Source: CAD feature listing. Evaluate the final solid. Frame: model axes, mm. A direction names the side the tool comes from. Give positions to 0.01 mm unless a question says otherwise; leave off trailing zeros. Order: outer loops, then holes, each group sorted by start corner. A loop starts at its lowest first (then second) coordinate and runs counter-clockwise, first axis right, second up. Notation, with made-up numbers: (46.5, 35) - (95.5, 35) arc R7 ccw to (95.5, 45) - close; hole circle Ø1 at (5.5, 49.5). An arc over 180 degrees is marked (long way). Write each question's results on one line, items separated by ' | '. Start each with the question number.
Item 1: Contact query for flat-ended pins moving along their axis: pin 1 Ø1 at (y, z) = (1.5, -3.5) entering from +X; pin 2 Ø6 at (x, y) = (-14.5, -3.5) entering from +Z; pin 3 Ø8 at (y, z) = (6.5, -5) entering from -X. Output: stop coordinate, or through.
Item 2: Mould query, pull axis Z, two halves, no side actions, for faces 4 (the flat face through (21.5, 2, -2)), 5 (the cylindrical face through (-31.584, 3.105, 1.615)), 6 (the cylindrical face through (0.52, -1.22, 0.27)). Classes: released by +Z, released by -Z, zero draft, split by the parting line, or undercut.
Item 3: Line query: line 1 along Y through (x, z) = (-10.5, 0); line 2 along X through (y, z) = (-4, 0); line 3 along Y through (x, z) = (-9, 1). Output: solid intervals per line, ascending.
Item 4: Set-up query: faces 1 (the cylindrical face through (20.49, -3.04, -3.32)), 2 (the flat face through (-37.5, 2, 0)), 3 (the flat face through (-25.5, 4, 0)). Return all of +Z, -Z, +X, -X, +Y, -Y with unobstructed straight access to the full face (end or side cutting, diameter ignored); none if empty.
Item 5: Section A-A on x = -3. Output: boundary loops of the cut face in (y, z).
Item 6: Section B-B on x = 23.5. Output: boundary loops of the cut face in (y, z), and give its area (3 significant figures).
```python
from build123d import *

# Parameters (mm, degrees)
REDONDEO1_R           = 2
CROQUIS2_R            = 1.25
CORTAR_EXTRUIR1_DEPTH = 76.944863877


with BuildPart() as part:
    # Croquis1 → Revolución1 (revolve)
    with BuildSketch(Plane.XY, mode=Mode.PRIVATE) as revoluci_n1_sk:
        with BuildLine():
            Line((-37.5, 0), (37.5, 0))
            Line((37.5, 0), (37.5, 2.5))
            Line((37.5, 2.5), (21.5, 2.5))
            Line((21.5, 2.5), (21.5, 4.5))
            Line((21.5, 4.5), (19.5, 4.5))
            ThreePointArc((19.5, 4.5), (11.232124598, 7.486529543), (2.5, 8.5))
            Line((2.5, 8.5), (2.5, 4.5))
            Line((2.5, 4.5), (-25.5, 4.5))
            Line((-25.5, 4.5), (-25.5, 3.5))
            Line((-25.5, 3.5), (-37.5, 3.5))
            Line((-37.5, 3.5), (-37.5, 0))
        make_face()
    revolve(revoluci_n1_sk.sketch.rotate(Axis((-37.5, 0, 0), (1, 0, 0)), 90), axis=Axis((-37.5, 0, 0), (1, 0, 0)))

    # Redondeo1
    redondeo1_edges = [part.edges().sort_by_distance(p)[0] for p in [
        (2.5, 0, -8.5),
    ]]
    fillet(redondeo1_edges, radius=REDONDEO1_R)

    # Croquis2 → Cortar-Extruir1 (cut, through all)
    with BuildSketch(Plane(origin=(37.5, 0, 0), x_dir=(0, 0, -1), z_dir=(1, 0, 0))):
        Circle(CROQUIS2_R)
    extrude(amount=-CORTAR_EXTRUIR1_DEPTH, mode=Mode.SUBTRACT)


solid = part.part
```
Evaluation:
1) pin 1: stops at x = 21.5 | pin 2: stops at z = 4.47 | pin 3: stops at x = -25.5
2) face 4: zero draft | face 5: split by the parting line | face 6: undercut
3) line 1: y = -4.5 to -1.25, 1.25 to 4.5 | line 2: x = -25.5 to 21.5 | line 3: y = -4.39 to -0.75, 0.75 to 4.39
4) face 1: +X | face 2: +Z, -Z, -X, +Y, -Y | face 3: -X
5) outline: circle Ø9 at (0, 0); hole circle Ø2.5 at (0, 0)
6) outline: circle Ø5 at (0, 0); hole circle Ø2.5 at (0, 0) | area: 14.7 mm^2
